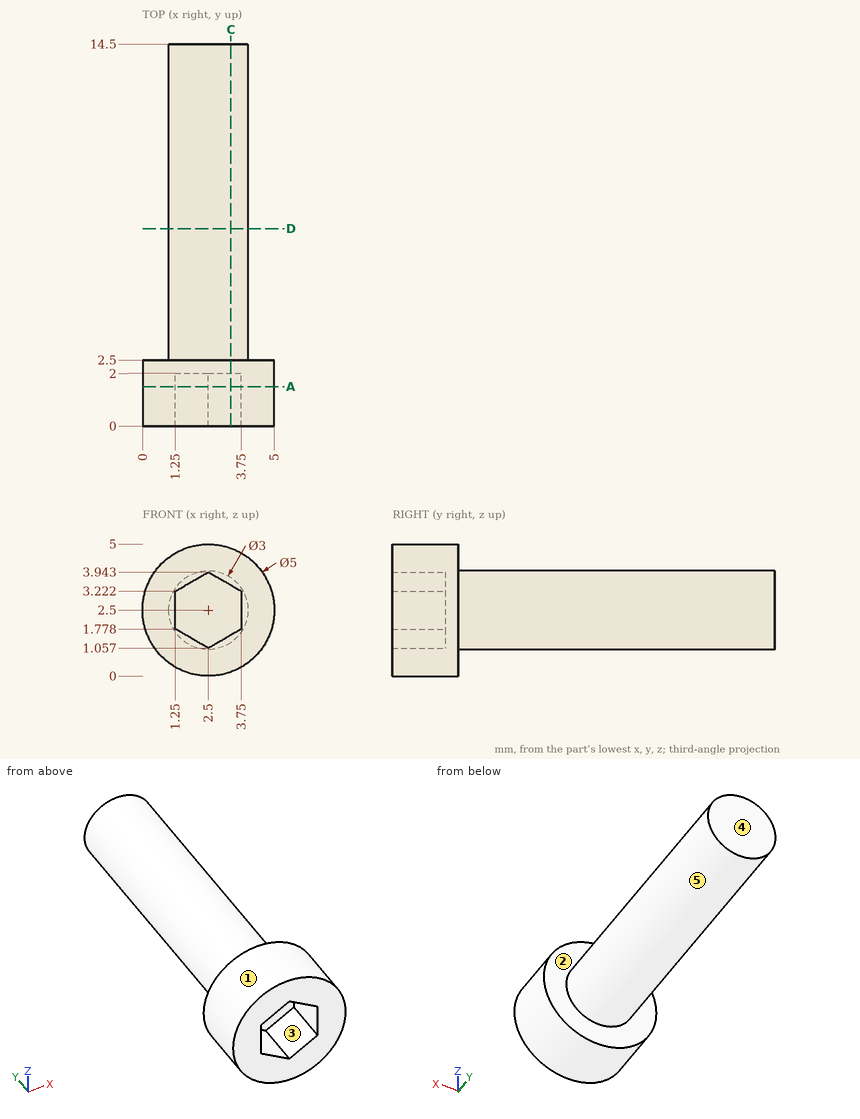
Job drawing, mm, ordinate dimensions from the low corner. One solid piece. A direction names the side the tool comes from. Give positions to 0.01 mm unless a question says otherwise; leave off trailing zeros. Loops run counter-clockwise (first coordinate to the right, second up) from the corner with the lowest first, then second, coordinate; pieces in that order, holes last. Notation, with made-up numbers: (-19.75, 83) - (8.25, 83) arc R26 cw to (8.25, 105) - close; hole circle Ø1 at (-16, 41.5). An arc over 180 degrees is marked (long way). Use one line per item in the form item = value.
(1) Drill centre lines: L1, parallel to Y at x = 3.95, z = 1.7; L2, parallel to X at y = 11.5, z = 2.55; L3, parallel to Z at x = 1.75, y = 1.5 (1 decimal). Where is each one in solid material? Low to high.
Determined:
L1 = 0 to 2.5
L2 = 1 to 4
L3 = 0.1 to 1.5, 3.5 to 4.9
(2) Drop flat-ended pins along their axis: P1, Ø2, axis at x = 3.5, y = 11.5, coming from the +Z side; P2, Ø0.8, axis at x = 2.5, z = 2, coming from the -Y side; P3, Ø1, axis at x = 3.5, z = 4.5, coming from the +Y side. Give the stop position or say it passes through.
Determined:
P1 = 4
P2 = 2
P3 = 2.5
(3) Cut at A-A (y = 1.5). Give the cut face in (x, z).
Determined:
outline = circle Ø5 at (2.5, 2.5); hole (1.25, 1.78) - (2.5, 1.06) - (3.75, 1.78) - (3.75, 3.22) - (2.5, 3.94) - (1.25, 3.22) - close
(4) Cut at C-C (x = 3.35). Give the cut face in (y, z), then the cut area to 3 significant figures.
Determined:
outline = (0, 0.15) - (2.5, 0.15) - (2.5, 1.26) - (14.5, 1.26) - (14.5, 3.74) - (2.5, 3.74) - (2.5, 4.85) - (0, 4.85) - (0, 3.45) - (2, 3.45) - (2, 1.55) - (0, 1.55) - close
area = 37.6 mm^2
(5) Cut at D-D (y = 7.5). Give the cut face in (x, z).
Determined:
outline = circle Ø3 at (2.5, 2.5)
(6) 3-axis set-ups, long thin cutter, end or side, ignore diameter. For the marked faces 1 and 2: which of +Z, -Z, +X, -X, +Y, -Y reach the whole face in a straight line?
Determined:
face_1 = +Y, -Y
face_2 = +Y
(7) Pull direction X, two halves, no side cores. Call the marked faces 3, 4 and 5: pulls with the +X half, pulls with the -X half, needs draft (parallel to the pull), parting line crosses it, or undercut.
Determined:
face_3 = undercut
face_4 = needs draft
face_5 = parting line crosses it
